Source: three-view drawing plus pictorial views. Frame: mm from the lowest corner of the part. A direction names the side the tool comes from. Give positions to 0.01 mm unless a question says otherwise; leave off trailing zeros. Order: outer loops, then holes, each group sorted by start corner. A loop starts at its lowest first (then second) coordinate and runs counter-clockwise, first axis right, second up. Notation, with made-up numbers: (42.5, 15) - (48.5, 15) arc R13 cw to (48.5, 32) - close; hole circle Ø1 at (66.25, -25). An arc over 180 degrees is marked (long way). Use one line per item in the form item = value.
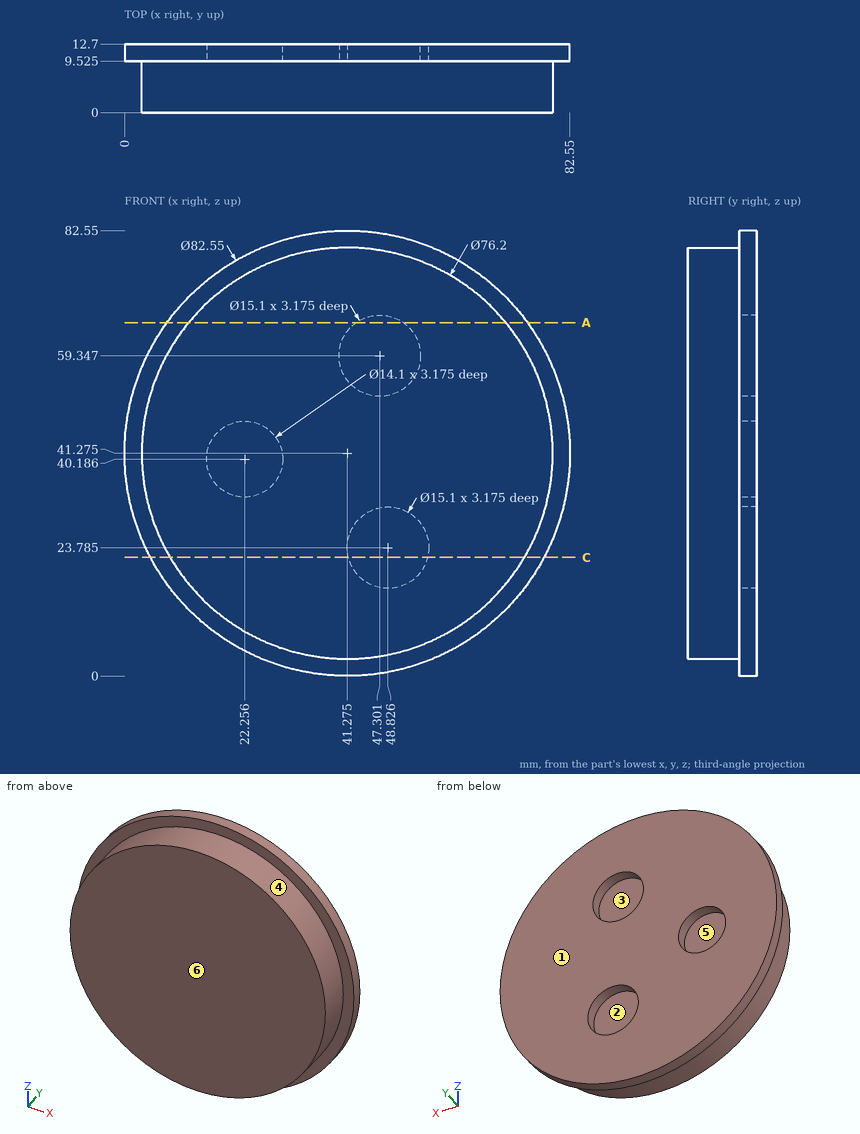
(1) Contact query for flat-ended pins moving along their axis: pin 1 Ø3 at (y, z) = (9.5, 62) entering from -X; pin 2 Ø8.5 at (x, z) = (22.26, 40.19) entering from +Y (3 decimals); pin 3 Ø3 at (x, y) = (33, 6.5) entering from -Z. Output: stop coordinate, or through.
Computed values:
pin_1 = 4.75
pin_2 = 9.525
pin_3 = 3.78
(2) Cut plane A-A on z = 65.5. Output: boundary loops of the cut face in (x, y) (1 decimal), plus the area to 3 significant figures.
Computed values:
outline = (7.9, 9.5) - (11.9, 9.5) - (11.9, 0) - (70.7, 0) - (70.7, 9.5) - (74.7, 9.5) - (74.7, 12.7) - (51.7, 12.7) - (51.7, 9.5) - (42.9, 9.5) - (42.9, 12.7) - (7.9, 12.7) - close
area = 745 mm²
(3) Ray query, line 1 along X through (y, z) = (11.75, 55.5) (1 decimal); line 2 along Z through (x, y) = (18, 12.25) (1 decimal); line 3 along X through (y, z) = (11.5, 35). Return the intervals inside material, ascending.
Computed values:
line_1 = 2.5 to 40.8, 53.8 to 80
line_2 = 7.2 to 34.6, 45.8 to 75.4
line_3 = 0.48 to 17.48, 27.03 to 82.07
(4) Reachability of the marked faces 1 and 2 from +Z, -Z, +X, -X, +Y, -Y: full face, straight path, thin tool, end or side. Return the list, or none.
Computed values:
face_1 = +Z, -Z, +X, -X, +Y
face_2 = +Y
(5) Cut plane C-C on z = 22. Output: boundary loops of the cut face in (x, y) (1 decimal).
Computed values:
outline = (4.8, 9.5) - (8.4, 9.5) - (8.4, 0) - (74.1, 0) - (74.1, 9.5) - (77.8, 9.5) - (77.8, 12.7) - (56.2, 12.7) - (56.2, 9.5) - (41.5, 9.5) - (41.5, 12.7) - (4.8, 12.7) - close
(6) Pull-direction query (X, two-part tool) for the marked faces 3, 4, 5 and 6; classes: released by +X, released by -X, zero draft, split by the parting line, or undercut.
Computed values:
face_3 = undercut
face_4 = split by the parting line
face_5 = undercut
face_6 = zero draft
